For this review, take the finished solid that the model builds, in its own axes (mm). A direction names the side the tool comes from. Give positions to 0.01 mm unless a question says otherwise; leave off trailing zeros. Loops run counter-clockwise (first coordinate to the right, second up) from the corner with the lowest first, then second, coordinate; pieces in that order, holes last. Notation, with made-up numbers: (45, -11.75) - (51, -11.75) arc R23 cw to (51, -1.75) - close; hole circle Ø1 at (9, 6.5). An arc over 180 degrees is marked (long way). Put each result on its own line as item: value. Start each with the question number.
from build123d import *

# Parameters (mm, degrees)
F0_R     = 11.5
F1_DEPTH = 10
F0_R_2   = 5
F2_DEPTH = 15


with BuildPart() as f1:
    # F0 (on Front) → F1 (new body)
    with BuildSketch(Plane.XZ):
        Polygon((0, 54), (0, 51.083995), (-9.377002, 53.179619), (-8.870643, 50.307914), (-18.469088, 50.743402), (-17.471755, 48.003253), (-27, 46.765372), (-25.541998, 44.240037), (-34.710531, 41.3664), (-32.836159, 39.132611), (-41.3664, 34.710531), (-39.132611, 32.836159), (-46.765372, 27), (-44.240037, 25.541998), (-50.743402, 18.469088), (-48.003253, 17.471755), (-53.179619, 9.377002), (-50.307914, 8.870643), (-54, 0), (-51.083995, 0), (-53.179619, -9.377002), (-50.307914, -8.870643), (-50.743402, -18.469088), (-48.003253, -17.471755), (-46.765372, -27), (-44.240037, -25.541998), (-41.3664, -34.710531), (-39.132611, -32.836159), (-34.710531, -41.3664), (-32.836159, -39.132611), (-27, -46.765372), (-25.541998, -44.240037), (-18.469088, -50.743402), (-17.471755, -48.003253), (-9.377002, -53.179619), (-8.870643, -50.307914), (0, -54), (0, -51.083995), (9.377002, -53.179619), (8.870643, -50.307914), (18.469088, -50.743402), (17.471755, -48.003253), (27, -46.765372), (25.541998, -44.240037), (34.710531, -41.3664), (32.836159, -39.132611), (41.3664, -34.710531), (39.132611, -32.836159), (46.765372, -27), (44.240037, -25.541998), (50.743402, -18.469088), (48.003253, -17.471755), (53.179619, -9.377002), (50.307914, -8.870643), (54, 0), (51.083995, 0), (53.179619, 9.377002), (50.307914, 8.870643), (50.743402, 18.469088), (48.003253, 17.471755), (46.765372, 27), (44.240037, 25.541998), (41.3664, 34.710531), (39.132611, 32.836159), (34.710531, 41.3664), (32.836159, 39.132611), (27, 46.765372), (25.541998, 44.240037), (18.469088, 50.743402), (17.471755, 48.003253), (9.377002, 53.179619), (8.870643, 50.307914), align=None)
        with BuildLine():
            Line((-6.683914, -9.966208), (-3.984963, -40.815351))
            ThreePointArc((-3.984963, -40.815351), (-5.242796, -43.506931), (-8.116223, -44.262026))
            ThreePointArc((-8.116223, -44.262026), (-31.813943, -31.825666), (-44.259032, -8.13253))
            ThreePointArc((-44.259032, -8.13253), (-43.505888, -5.259895), (-40.816663, -4))
            Line((-40.816663, -4), (-9.129554, -7.524517))
            ThreePointArc((-9.129554, -7.524517), (-7.741489, -8.57985), (-6.683914, -9.966208))
        make_face(mode=Mode.SUBTRACT)
        with BuildLine():
            Line((9.966208, -6.683914), (40.815351, -3.984963))
            ThreePointArc((40.815351, -3.984963), (43.506931, -5.242796), (44.262026, -8.116223))
            ThreePointArc((44.262026, -8.116223), (31.825666, -31.813943), (8.13253, -44.259032))
            ThreePointArc((8.13253, -44.259032), (5.259895, -43.505888), (4, -40.816663))
            Line((4, -40.816663), (7.524517, -9.129554))
            ThreePointArc((7.524517, -9.129554), (8.57985, -7.741489), (9.966208, -6.683914))
        make_face(mode=Mode.SUBTRACT)
        with BuildLine():
            ThreePointArc((-44.262026, 8.116223), (-31.825666, 31.813943), (-8.13253, 44.259032))
            ThreePointArc((-8.13253, 44.259032), (-5.259895, 43.505888), (-4, 40.816663))
            Line((-4, 40.816663), (-7.524517, 9.129554))
            ThreePointArc((-7.524517, 9.129554), (-8.57985, 7.741489), (-9.966208, 6.683914))
            Line((-9.966208, 6.683914), (-40.815351, 3.984963))
            ThreePointArc((-40.815351, 3.984963), (-43.506931, 5.242796), (-44.262026, 8.116223))
        make_face(mode=Mode.SUBTRACT)
        Circle(F0_R, mode=Mode.SUBTRACT)
        with BuildLine():
            Line((6.683914, 9.966208), (3.984963, 40.815351))
            ThreePointArc((3.984963, 40.815351), (5.242796, 43.506931), (8.116223, 44.262026))
            ThreePointArc((8.116223, 44.262026), (31.813943, 31.825666), (44.259032, 8.13253))
            ThreePointArc((44.259032, 8.13253), (43.505888, 5.259895), (40.816663, 4))
            Line((40.816663, 4), (9.129554, 7.524517))
            ThreePointArc((9.129554, 7.524517), (7.741489, 8.57985), (6.683914, 9.966208))
        make_face(mode=Mode.SUBTRACT)
    extrude(amount=-F1_DEPTH)

    # F0 (on Front) → F2 (join)
    with BuildSketch(Plane.XZ):
        Circle(F0_R)
        Circle(F0_R_2, mode=Mode.SUBTRACT)
    extrude(amount=-F2_DEPTH)


solid = f1.part
1) Machinability: for faces 5 (the flat face through (-29.959, 4.93, -42.896)), 6 (the flat face through (-47.446, 4.93, 22.055)), 7 (the flat face through (5.353, 4.93, 25.175)), which of the approach directions +Z, -Z, +X, -X, +Y, -Y give a long, thin tool a straight path to every point of the face, cutting with its end or side? Answer none if there is none.
2) Take a section at B-B on x = 36. State the section outline as (y, z) points, and give its area (3 significant figures).
3) Mouldability with a two-part tool opening along Z and no side actions: class faces 1 (the flat face through (-17.977, 4.93, -49.393)), 2 (the flat face through (25.175, 4.93, -5.353)), 3 (the flat face through (53, 5, 0)), 4 (the flat face through (-4.623, 4.93, 52.117)) as released by +Z, released by -Z, zero draft, split by the parting line, or undercut.
4) Wall thickness on probe 1 along Z at (x, y) = (-19, 0.75); probe 2 along X at (y, z) = (4, 25); probe 3 along Z at (x, y) = (35, 8): over which ranges is each line inside the solid? List them lowest first.
5) Insertion check: P1, Ø0.9, axis at x = 53, y = 3.5, coming from the +Z side; P2, Ø3, axis at x = -35, z = 43, coming from the -Y side; P3, Ø6, axis at y = 6, z = -10, coming from the -X side; P4, Ø2.5, axis at y = 6, z = -53, coming from the +X side. Each pin has a flat end and moves straight along its axis. Give the tip position at first contact, or say it passes through.
6) Take a section at A-A on z = -24. State the section outline as (x, y) points, and give its area (3 significant figures).
Answers follow:
1. face 5: -Z, +Y, -Y
1. face 6: -X, +Y, -Y
1. face 7: +Y, -Y
2. outline: (0, -37.49) - (10, -37.49) - (10, -27) - (0, -27) - close; (0, -4.41) - (10, -4.41) - (10, 4.54) - (0, 4.54) - close; (0, 27) - (10, 27) - (10, 38.88) - (0, 38.88) - close
2. area: 313 mm2
3. face 1: released by -Z
3. face 2: undercut
3. face 3: undercut
3. face 4: released by +Z
4. probe 1: -50.26 to -40.79, -6.43 to 5.89, 40.79 to 47.8
4. probe 2: -44.74 to -37.42, -5.76 to 5.37, 37.42 to 47.03
4. probe 3: -38.01 to -28.28, -4.49 to 4.65, 28.28 to 40.81
5. P1: z = 9.38
5. P2: through
5. P3: x = -53.18
5. P4: x = 9.38
6. outline: (-47.16, 0) - (-38.07, 0) - (-38.07, 10) - (-47.16, 10) - close; (-5.46, 0) - (5.87, 0) - (5.87, 10) - (-5.46, 10) - close; (38.07, 0) - (45.66, 0) - (45.66, 10) - (38.07, 10) - close
6. area: 280 mm2
